```python
from build123d import *

# Parameters (mm, degrees)
F1_R     = 8.15
F1_R_2   = 6.95
F3_R     = 3
F4_DEPTH = 12.5
F5_R     = 3.3
F6_DEPTH = 12.5


with BuildPart() as f2:
    # F2: sweep along a path in F0
    with BuildLine(Plane.XZ) as f2_path:
        Line((0, 0), (-35, 0))
        ThreePointArc((-35, 0), (-64.6984848098, 12.3015151902), (-77, 42))
        Line((-77, 42), (-77, 207))
    # F1 (on Right) → F2 (sweep)
    with BuildSketch(Plane.YZ):
        Circle(F1_R)
        Circle(F1_R_2, mode=Mode.SUBTRACT)
    sweep(path=f2_path.line)

    # F3 (on Front) → F4 (cut, symmetric)
    with BuildSketch(Plane.XZ):
        with Locations((-64.6984848098, 12.3015151902)):
            Circle(F3_R)
    extrude(amount=F4_DEPTH, both=True, mode=Mode.SUBTRACT)

    # F5 (on Top) → F6 (cut, symmetric)
    with BuildSketch(Plane.XY):
        with Locations((-9.9, 0)):
            Circle(F5_R)
    extrude(amount=F6_DEPTH, both=True, mode=Mode.SUBTRACT)


solid = f2.part
```
For this review, take the finished solid that the model builds, in its own axes (mm). A direction names the side the tool comes from. Round coordinates to 2 decimals unless told otherwise and drop trailing zeros. Write each loop counter-clockwise with the first axis right and the second up, starting at its lowest first coordinate (ties: lowest second). Pieces come first, ordered by that corner, then holes. Notation, with made-up numbers: (53, 53.5) -> (78, 53.5) arc R12 ccw to (78, 60.5) -> close; hole circle Ø9 at (43, 6.5). An arc over 180 degrees is marked (long way). One line per question, with ' | ' between items. Start each with the question number.
1) Add section C-C (x = -18). Write out the cut boundary in (y, z), and give its area (3 significant figures).
2) Wall thickness on line 1 along Y through (x, z) = (-77, 146); line 2 along X through (y, z) = (-5, 76): over which ranges is each line inside the solid? List them lowest first.
3) For pin 1 Ø1.5 at (y, z) = (6, 127) entering from -X; pin 2 Ø1.5 at (x, z) = (-69, 172) entering from +Y; pin 3 Ø1.5 at (x, y) = (-17.5, -1) entering from -Z, all flat-tipped, find the tip position at first contact; note any pin that passes through.
4) Add section B-B (z = 60.5). Write out the cut boundary in (x, y).
5) Mouldability with a two-part tool opening along X and no side actions: class faces 1 (the cylindrical face through (-66.91, -7.22, 14.33)), 2 (the cylindrical face through (-69.77, 3.76, 125.66)), 3 (the flat face through (-83, 4, 207)) as +X half, -X half, draft (parallel to the pull), parting line (faces both ways), or undercut.
6) Add section A-A (y = 0). Write out the cut boundary in (x, z).
7) Machinability: for faces 4 (the cylindrical face through (-66.91, 7.19, 14.33)), 5 (the cylindrical face through (-82.86, 3.74, 125.66)), 6 (the cylindrical face through (-17.745, 7.774, -2.448)), which of the approach directions +Z, -Z, +X, -X, +Y, -Y give a long, thin tool a straight path to every point of the face, cutting with its end or side? Answer none if there is none.
Reported:
1) outline: circle Ø16.3 at (0, 0); hole circle Ø13.9 at (0, 0) | area: 56.9 mm²
2) line 1: y = -8.15 to -6.95, 6.95 to 8.15 | line 2: x = -83.44 to -81.83, -72.17 to -70.56
3) pin 1: stops at x = -83.23 | pin 2: stops at y = 3.72 | pin 3: stops at z = -8.15
4) outline: circle Ø16.3 at (-77, 0); hole circle Ø13.9 at (-77, 0)
5) face 1: undercut | face 2: parting line | face 3: draft
6) outline: (-85.15, 42) arc R50.15 ccw to (-35, -8.15) -> (-13.2, -8.15) -> (-13.2, -6.95) -> (-35, -6.95) arc R48.95 cw to (-83.95, 42) -> (-83.95, 207) -> (-85.15, 207) -> close; (-70.05, 42) arc R35.05 ccw to (-35, 6.95) -> (-13.2, 6.95) -> (-13.2, 8.15) -> (-35, 8.15) arc R33.85 cw to (-68.85, 42) -> (-68.85, 207) -> (-70.05, 207) -> close; (-6.6, -8.15) -> (0, -8.15) -> (0, -6.95) -> (-6.6, -6.95) -> close; (-6.6, 6.95) -> (0, 6.95) -> (0, 8.15) -> (-6.6, 8.15) -> close
7) face 4: +Y, -Y | face 5: +Z | face 6: +X
